The model under review builds one solid part; all positions refer to its coordinate system, in mm. Round coordinates to 2 decimals unless told otherwise and drop trailing zeros. Loops run counter-clockwise (first coordinate to the right, second up) from the corner with the lowest first, then second, coordinate; pieces in that order, holes last. Notation, with made-up numbers: (-25, 22.25) -> (-8, 22.25) arc R10 cw to (-8, 32.25) -> close; hole circle Ø8 at (76, -30.5). An arc over 180 degrees is marked (long way). Return JSON: item names as keys, results as strings. Group by question number.
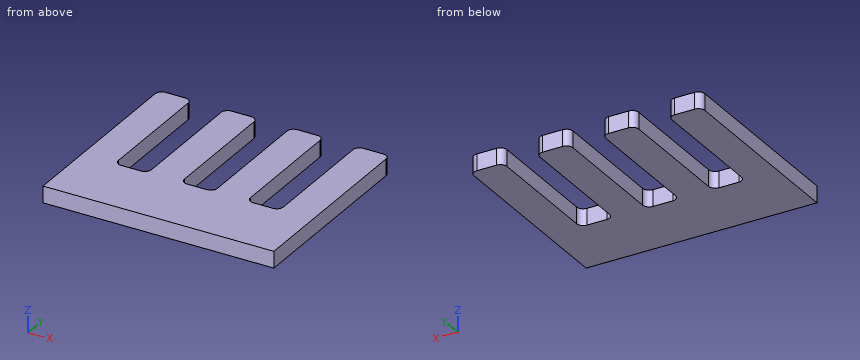
```python
from build123d import *

# Parameters (mm, degrees)
F1_DEPTH = 5
F2_R     = 2


with BuildPart() as f1:
    # F0 (on Top) → F1 (new body)
    with BuildSketch(Plane.XY):
        Polygon((0, 60), (0, 0), (70, 0), (70, 60), (60, 60), (60, 20), (50, 20), (50, 60), (40, 60), (40, 20), (30, 20), (30, 60), (20, 60), (20, 20), (10, 20), (10, 60), align=None)
    extrude(amount=F1_DEPTH)

    # F2
    f2_edges = [f1.edges().sort_by_distance(p)[0] for p in [
        (10, 60, 2.5),
        (0, 60, 2.5),
        (20, 60, 2.5),
        (30, 60, 2.5),
        (40, 60, 2.5),
        (50, 60, 2.5),
        (60, 60, 2.5),
        (70, 60, 2.5),
        (10, 20, 2.5),
        (20, 20, 2.5),
        (30, 20, 2.5),
        (40, 20, 2.5),
        (50, 20, 2.5),
        (60, 20, 2.5),
    ]]
    fillet(f2_edges, radius=F2_R)


solid = f1.part
```
1. We need section C-C, the plane x = 17. Write out the cut boundary in (y, z), then the cut area to 3 significant figures.
2. Wall thickness on line 1 (X direction, y = 56.5, z = 4.3); line 2 (Y direction, x = 16.5, z = 3.95); line 3 (Y direction, x = 19, z = 0.9): over which ranges is each line inside the solid? List them lowest first.
3. We need section A-A, the plane y = 36. Write out the cut boundary in (x, z).
4. For P1, Ø1.5, axis at x = 36.5, z = 3.5, coming from the +Y side, flat-tipped, find the tip position at first contact; note if it passes through.
Check sheet entries:
{
 "1": {"outline": "(0, 0) -> (20, 0) -> (20, 5) -> (0, 5) -> close", "area": "100 mm²"},
 "2": {"line 1": "x = 0 to 10, 20 to 30, 40 to 50, 60 to 70", "line 2": "y = 0 to 20", "line 3": "y = 0 to 20.27"},
 "3": {"outline": "(0, 0) -> (10, 0) -> (10, 5) -> (0, 5) -> close; (20, 0) -> (30, 0) -> (30, 5) -> (20, 5) -> close; (40, 0) -> (50, 0) -> (50, 5) -> (40, 5) -> close; (60, 0) -> (70, 0) -> (70, 5) -> (60, 5) -> close"},
 "4": {"P1": "stops at y = 20"}
}
